Drawing for the job (mm, zero at the part's lowest x, y, z). A direction names the side the tool comes from. Coordinates: 2 decimals unless noted, no trailing zeros. Write each loop counter-clockwise with the first axis right and the second up, starting at its lowest first coordinate (ties: lowest second). Pieces come first, ordered by that corner, then holes. Notation, with made-up numbers: (51, 86) -> (97, 86) arc R38 ccw to (97, 124) -> close; hole circle Ø11 at (-14, 56). An arc over 180 degrees is marked (long way). Write item = value, one per line. Start each with the question number.
Q1. Band-saw the part on C-C, the plane x = 17. List the corners of the cut face in (y, z).
Q2. Tool access for the marked faces 1, 2 and 3: list every direction of +Z, -Z, +X, -X, +Y, -Y with a clear straight run to the whole face (end or side of a thin tool).
Q3. Probe line 1 (Y direction, x = 15.5, z = 3.45); line 2 (Y direction, x = 11.5, z = 0.7); line 3 (X direction, y = 9.25, z = 1.75). List the from-to ranges inside material, lowest first.
Q4. Pin check, flat tips, straight feed: P1, Ø0.9, axis at x = 8, z = 3, coming from the +Y side; P2, Ø1.5, axis at x = 8, z = 2.5, coming from the -Y side; P3, Ø1.5, axis at y = 7.5, z = 2.5, coming from the -X side. Stop position of each tip, or through.
Q5. Band-saw the part on B-B, the plane z = 3.05. List the corners of the cut face in (x, y), plus the area to 3 significant figures.
Q6. Pull direction Y, two halves, no side cores. Call the marked faces 4, 5 and 6: released by +Y, released by -Y, zero draft, split by the parting line, or undercut.
Q7. Band-saw the part on A-A, the plane y = 8.25. List the corners of the cut face in (x, z), plus the area to 3 significant figures.
Q8. Band-saw the part on D-D, the plane x = 20.25. List the corners of the cut face in (y, z), plus the area to 3 significant figures.
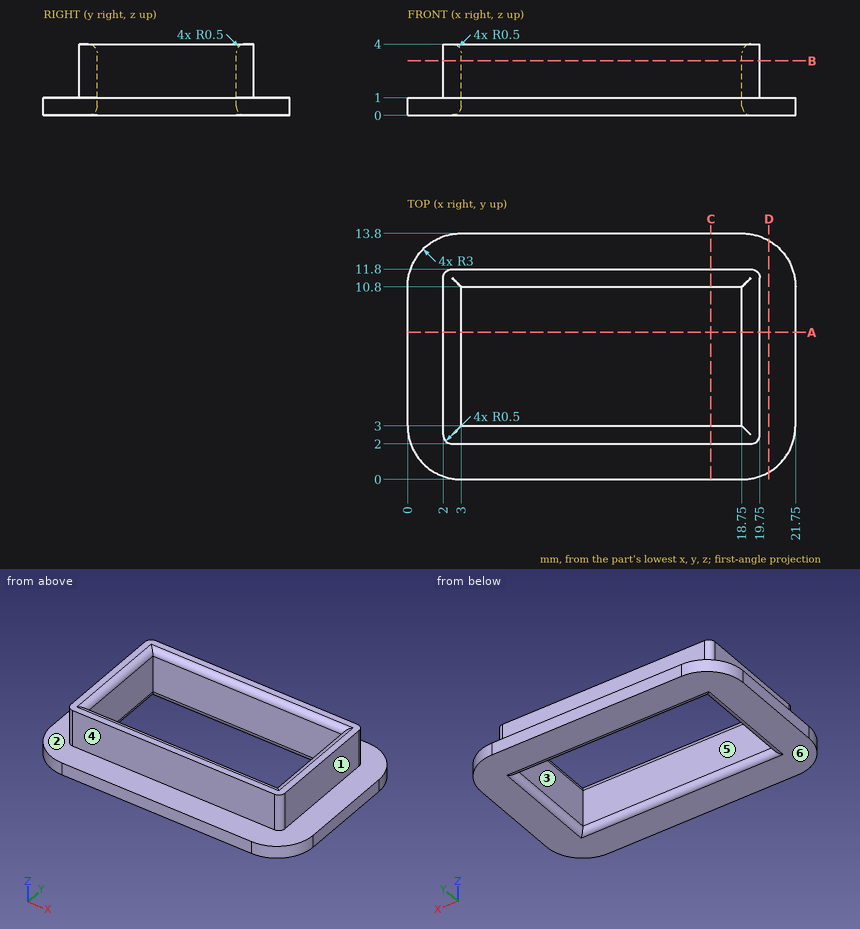
Ans:
q1.outline = (0, 0) -> (2.5, 0) arc R0.5 ccw to (3, 0.5) -> (3, 3.5) arc R0.5 ccw to (2.5, 4) -> (2, 4) -> (2, 1) -> (0, 1) -> close; (10.8, 0.5) arc R0.5 ccw to (11.3, 0) -> (13.8, 0) -> (13.8, 1) -> (11.8, 1) -> (11.8, 4) -> (11.3, 4) arc R0.5 ccw to (10.8, 3.5) -> close
q2.face_1 = +Z, +X, +Y, -Y
q2.face_2 = +Z
q2.face_3 = +Z, -Z
q3.line_1 = 2 to 3, 10.8 to 11.8
q3.line_2 = 0 to 3, 10.8 to 13.8
q3.line_3 = 2 to 3, 18.75 to 19.75
q4.P1 = 11.8
q4.P2 = 2
q4.P3 = 2
q5.outline = (2, 2.5) arc R0.5 ccw to (2.5, 2) -> (19.25, 2) arc R0.5 ccw to (19.75, 2.5) -> (19.75, 11.3) arc R0.5 ccw to (19.25, 11.8) -> (2.5, 11.8) arc R0.5 ccw to (2, 11.3) -> close; hole (3, 3) -> (18.75, 3) -> (18.75, 10.8) -> (3, 10.8) -> close
q5.area = 50.9 mm2
q6.face_4 = released by -Y
q6.face_5 = undercut
q6.face_6 = zero draft
q7.outline = (0, 0) -> (2.5, 0) arc R0.5 ccw to (3, 0.5) -> (3, 3.5) arc R0.5 ccw to (2.5, 4) -> (2, 4) -> (2, 1) -> (0, 1) -> close; (18.75, 0.5) arc R0.5 ccw to (19.25, 0) -> (21.75, 0) -> (21.75, 1) -> (19.75, 1) -> (19.75, 4) -> (19.25, 4) arc R0.5 ccw to (18.75, 3.5) -> close
q7.area = 11.8 mm2
q8.outline = (0.4, 0) -> (13.4, 0) -> (13.4, 1) -> (0.4, 1) -> close
q8.area = 13.0 mm2
